Check sheet for the modelled part. Datum: model origin and axes. Units: mm. Face numbers are marked on the shaded views. A direction names the side the tool comes from. Give positions to 0.01 mm unless a question says otherwise; leave off trailing zeros. Order: outer loops, then holes, each group sorted by start corner. A loop starts at its lowest first (then second) coordinate and runs counter-clockwise, first axis right, second up.
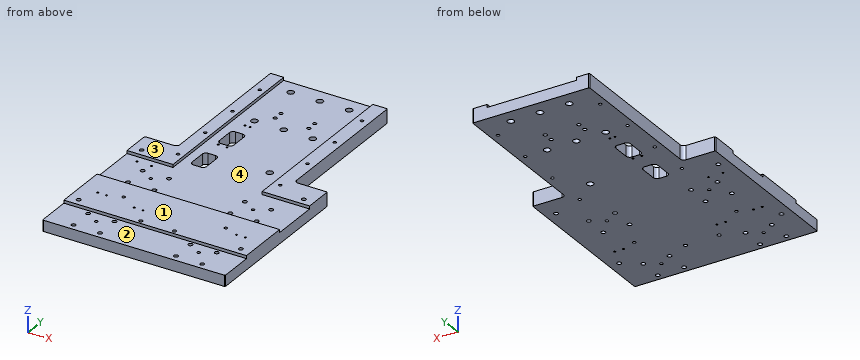
```python
from build123d import *

# Parameters (mm, degrees)
BOSS_EXTRUDE1_DEPTH   = 19.05
SKETCH2_W             = 250
SKETCH2_H             = 47
CUT_EXTRUDE1_DEPTH    = 4.05
M5_CLEARANCE_HOLE2_D  = 5.8
M5_CLEARANCE_HOLE1_D  = 5.8
M5X0_8_TAPPED_HOLE1_D = 4.2
LPATTERN1_COUNT       = 7
LPATTERN1_PITCH       = 60
MIRROR2_COPY_1_D      = 5.8
MIRROR2_COPY_2_D      = 4.2
MIRROR2_COPY_3_D      = 4.2
MIRROR2_COPY_4_D      = 4.2
MIRROR2_COPY_5_D      = 4.2
MIRROR2_COPY_6_D      = 4.2
MIRROR2_COPY_7_D      = 4.2
M8_CLEARANCE_HOLE1_D  = 9
M6X1_0_TAPPED_HOLE2_D = 5
M3X0_5_TAPPED_HOLE3_D = 2.5
M3X0_5_TAPPED_HOLE1_D = 2.5
M3X0_5_TAPPED_HOLE2_D = 2.5
CUT_EXTRUDE2_REACH    = 369.253
M3X0_5_TAPPED_HOLE4_D = 2.5
FILLET1_R             = 5
CHAMFER1_SIZE         = 1


with BuildPart() as part:
    # Sketch1 → Boss-Extrude1 (new body)
    with BuildSketch(Plane.XY):
        Polygon((-125, 140), (-125, -85), (125, -85), (125, 140), (80, 140), (80, 345), (-80, 345), (-80, 140), align=None)
    extrude(amount=BOSS_EXTRUDE1_DEPTH)

    # Sketch2 → Cut-Extrude1 (cut)
    with BuildSketch(Plane.XY.offset(19.05)):
        with Locations((0, -61.5)):
            Rectangle(SKETCH2_W, SKETCH2_H)
        Polygon((-125, 35), (125, 35), (125, 101), (60, 101), (60, 345), (-62, 345), (-62, 101), (-125, 101), align=None)
    extrude(amount=-CUT_EXTRUDE1_DEPTH, mode=Mode.SUBTRACT)

    # M5 Clearance Hole2 (through all)
    with Locations(Plane.XY.offset(15)):
        with Locations((-88, 76), (-52, 76), (-52, 44), (-88, 44)):
            m5_clearance_hole2 = Hole(M5_CLEARANCE_HOLE2_D / 2)

    # Mirror1: M5 Clearance Hole2 across plane
    add(m5_clearance_hole2.mirror(Plane.ZX), mode=Mode.SUBTRACT)

    # M5 Clearance Hole1 (through all)
    with Locations(Plane.XY.offset(19.05)):
        with Locations((-111, 111), (-111, -28)):
            m5_clearance_hole1 = Hole(M5_CLEARANCE_HOLE1_D / 2)

    # M5x0.8 Tapped Hole1 (through all)
    with Locations(Plane.XY.offset(19.05)):
        with Locations((-70, -55)):
            m5x0_8_tapped_hole1 = Hole(M5X0_8_TAPPED_HOLE1_D / 2)

    # LPattern1: M5x0.8 Tapped Hole1 ×7
    with Locations(*[(0, i * LPATTERN1_PITCH, 0) for i in range(1, LPATTERN1_COUNT)]):
        add(m5x0_8_tapped_hole1, mode=Mode.SUBTRACT)

    # Mirror2: M5 Clearance Hole2, M5 Clearance Hole1, M5x0.8 Tapped Hole1 across plane
    add(m5_clearance_hole2.mirror(Plane(origin=(0, 0, 0), x_dir=(0, 0, 1), z_dir=(1, 0, 0))), mode=Mode.SUBTRACT)
    add(m5_clearance_hole1.mirror(Plane(origin=(0, 0, 0), x_dir=(0, 0, 1), z_dir=(1, 0, 0))), mode=Mode.SUBTRACT)
    add(m5x0_8_tapped_hole1.mirror(Plane(origin=(0, 0, 0), x_dir=(0, 0, 1), z_dir=(1, 0, 0))), mode=Mode.SUBTRACT)

    # Mirror2 copy 1 (through all)
    with Locations(Plane(origin=(0, 0, 15), x_dir=(-1, 0, 0), z_dir=(0, 0, 1))):
        with Locations((-88, 76), (-52, 76), (-52, 44), (-88, 44)):
            Hole(MIRROR2_COPY_1_D / 2)

    # Mirror2 copy 2 (through all)
    with Locations(Plane(origin=(0, 60, 19.05), x_dir=(-1, 0, 0), z_dir=(0, 0, 1))):
        with Locations((-70, 55)):
            Hole(MIRROR2_COPY_2_D / 2)

    # Mirror2 copy 3 (through all)
    with Locations(Plane(origin=(0, 120, 19.05), x_dir=(-1, 0, 0), z_dir=(0, 0, 1))):
        with Locations((-70, 55)):
            Hole(MIRROR2_COPY_3_D / 2)

    # Mirror2 copy 4 (through all)
    with Locations(Plane(origin=(0, 180, 19.05), x_dir=(-1, 0, 0), z_dir=(0, 0, 1))):
        with Locations((-70, 55)):
            Hole(MIRROR2_COPY_4_D / 2)

    # Mirror2 copy 5 (through all)
    with Locations(Plane(origin=(0, 240, 19.05), x_dir=(-1, 0, 0), z_dir=(0, 0, 1))):
        with Locations((-70, 55)):
            Hole(MIRROR2_COPY_5_D / 2)

    # Mirror2 copy 6 (through all)
    with Locations(Plane(origin=(0, 300, 19.05), x_dir=(-1, 0, 0), z_dir=(0, 0, 1))):
        with Locations((-70, 55)):
            Hole(MIRROR2_COPY_6_D / 2)

    # Mirror2 copy 7 (through all)
    with Locations(Plane(origin=(0, 360, 19.05), x_dir=(-1, 0, 0), z_dir=(0, 0, 1))):
        with Locations((-70, 55)):
            Hole(MIRROR2_COPY_7_D / 2)

    # M8 Clearance Hole1 (through all)
    with Locations(Plane.XY.offset(15)):
        with Locations((-40, 325), (40, 325), (40, 245), (40, 150), (-40, 245), (0, 325), (0, 245)):
            Hole(M8_CLEARANCE_HOLE1_D / 2)

    # M6x1.0 Tapped Hole2 (through all)
    with Locations(Plane.XY.offset(19.05)):
        with Locations((-23, 276.5), (23, 263.5), (-23, 263.5), (23, 276.5), (-23, -32.5), (23, -32.5)):
            Hole(M6X1_0_TAPPED_HOLE2_D / 2)

    # M3x0.5 Tapped Hole3 (through all)
    with Locations(Plane.XY.offset(19.05)):
        with Locations((-101, -2), (-89, -2), (89, -2), (101, -2)):
            Hole(M3X0_5_TAPPED_HOLE3_D / 2)

    # M3x0.5 Tapped Hole1 (through all)
    with Locations(Plane.XY.offset(15)):
        with Locations((-105, 91), (-85, 91)):
            Hole(M3X0_5_TAPPED_HOLE1_D / 2)

    # M3x0.5 Tapped Hole2 (through all)
    with Locations(Plane(origin=(0, 0, 0), x_dir=(1, 0, 0), z_dir=(0, 0, -1))):
        with Locations((-43.5, -230), (-36.5, -230)):
            Hole(M3X0_5_TAPPED_HOLE2_D / 2)

    # Sketch20 → Cut-Extrude2 (cut, up to next)
    with BuildSketch(Plane.XY.offset(15), mode=Mode.PRIVATE) as cut_extrude2_sk1:
        with BuildLine():
            Line((-50, 206.25), (-50, 183.75))
            ThreePointArc((-50, 183.75), (-48.535533906, 180.214466094), (-45, 178.75))
            Line((-45, 178.75), (-35, 178.75))
            ThreePointArc((-35, 178.75), (-31.464466094, 180.214466094), (-30, 183.75))
            Line((-30, 183.75), (-30, 206.25))
            ThreePointArc((-30, 206.25), (-31.464466094, 209.785533906), (-35, 211.25))
            Line((-35, 211.25), (-45, 211.25))
            ThreePointArc((-45, 211.25), (-48.535533906, 209.785533906), (-50, 206.25))
        make_face()
    cut_extrude2_tool1 = extrude(cut_extrude2_sk1.sketch, amount=-CUT_EXTRUDE2_REACH, mode=Mode.PRIVATE) & part.part
    # Sketch20 → Cut-Extrude2 (cut, up to next)
    with BuildSketch(Plane.XY.offset(15), mode=Mode.PRIVATE) as cut_extrude2_sk2:
        with BuildLine():
            Line((-50, 146.25), (-50, 123.75))
            ThreePointArc((-50, 123.75), (-48.535533906, 120.214466094), (-45, 118.75))
            Line((-45, 118.75), (-35, 118.75))
            ThreePointArc((-35, 118.75), (-31.464466094, 120.214466094), (-30, 123.75))
            Line((-30, 123.75), (-30, 146.25))
            ThreePointArc((-30, 146.25), (-31.464466094, 149.785533906), (-35, 151.25))
            Line((-35, 151.25), (-45, 151.25))
            ThreePointArc((-45, 151.25), (-48.535533906, 149.785533906), (-50, 146.25))
        make_face()
    cut_extrude2_tool2 = extrude(cut_extrude2_sk2.sketch, amount=-CUT_EXTRUDE2_REACH, mode=Mode.PRIVATE) & part.part
    add(cut_extrude2_tool1.solids().sort_by_distance((-40, 195, 15))[0], mode=Mode.SUBTRACT)
    add(cut_extrude2_tool2.solids().sort_by_distance((-40, 135, 15))[0], mode=Mode.SUBTRACT)

    # M3x0.5 Tapped Hole4 (through all)
    with Locations(Plane(origin=(0, 0, 0), x_dir=(-1, 0, 0), z_dir=(0, 0, -1))):
        with Locations((34, 175), (46, 175), (34, -10), (46, -10)):
            Hole(M3X0_5_TAPPED_HOLE4_D / 2)

    # Fillet1
    fillet1_edges = [part.edges().sort_by_distance(p)[0] for p in [
        (-80, 140, 9.525),
        (80, 140, 9.525),
    ]]
    fillet(fillet1_edges, radius=FILLET1_R)

    # Chamfer1
    chamfer1_edges = [part.edges().sort_by_distance(p)[0] for p in [
        (-80, 345, 9.525),
        (80, 345, 9.525),
        (125, 140, 9.525),
        (-125, 140, 9.525),
        (125, -85, 7.5),
        (-125, -85, 7.5),
    ]]
    chamfer(chamfer1_edges, length=CHAMFER1_SIZE)


solid = part.part
```
(1) Set-up check for the marked faces 1 and 2: record each of +Z, -Z, +X, -X, +Y, -Y from which the full face is reachable in a straight line by a thin tool's end or side.
Response values:
face 1: +Z, +X, -X, +Y, -Y
face 2: +Z, +X, -X, -Y
(2) Release check for a two-part mould opening along Y. For the marked faces 3 and 4 record: released by +Y, released by -Y, zero draft, split by the parting line, or undercut.
Response values:
face 3: zero draft
face 4: undercut
(3) Cross-section at A-A on x = -0.5. Enter the section's corners in (y, z).
Response values:
outline: (-85, 0) - (240.53, 0) - (240.53, 15) - (35, 15) - (35, 19.05) - (-38, 19.05) - (-38, 15) - (-85, 15) - close; (249.47, 0) - (320.53, 0) - (320.53, 15) - (249.47, 15) - close; (329.47, 0) - (345, 0) - (345, 15) - (329.47, 15) - close
(4) Gauge pin test, flat ends, axial feed: pin 1 Ø6.5 at (x, y) = (88, 76) entering from +Z; pin 2 Ø3.5 at (x, y) = (88, 44) entering from +Z; pin 3 Ø2 at (y, z) = (234, 11) entering from -X; pin 4 Ø3 at (x, z) = (11.5, 17.5) entering from +Y. Record the tip position at first contact, or that the pin passes through.
Response values:
pin 1: stops at z = 15
pin 2: passes through
pin 3: stops at x = -80
pin 4: stops at y = 35
(5) Material ranges on L1, parallel to X at y = 263.5, z = 6.75; L2, parallel to Y at x = 40, z = 4; L3, parallel to X at y = 273, z = 16, recorded low to high.
Response values:
L1: x = -80 to -25.5, -20.5 to 20.5, 25.5 to 80
L2: y = -85 to 145.5, 154.5 to 240.5, 249.5 to 320.5, 329.5 to 345
L3: x = -80 to -62, 60 to 80
(6) Cross-section at B-B on z = 7. Count the separate pieces of the cut face and the enclosed holes in it, then the cut area to 3 significant figures.
Response values:
separate pieces: 1
enclosed holes: 61
area: 86,500 mm2
